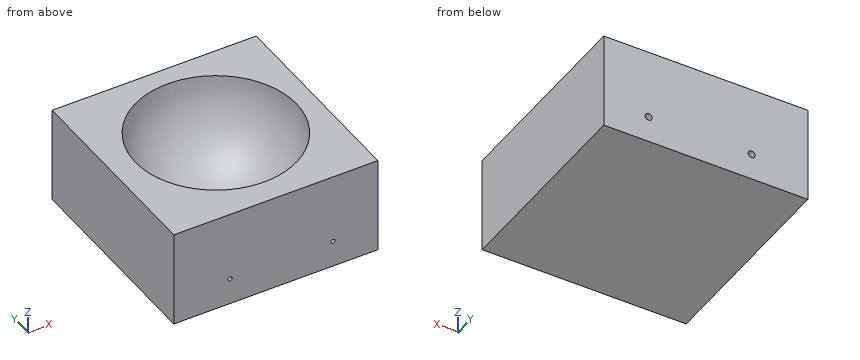
```python
from build123d import *

# Parameters (mm, degrees)
F0_W           = 190
F0_H           = 190
F1_DEPTH       = 90
F5_D           = 4
F5_CBORE_D     = 6.5
F5_CBORE_DEPTH = 50


with BuildPart() as f1:
    # F0 (on Top) → F1 (new body)
    with BuildSketch(Plane.XY):
        with Locations((-2.279991, -2.496977)):
            Rectangle(F0_W, F0_H)
    extrude(amount=F1_DEPTH)

    # F2 (on face) → F3 (revolve, cut)
    with BuildSketch(Plane.XY.offset(90)):
        with BuildLine():
            Line((75, 0), (-75, 0))
            ThreePointArc((-75, 0), (0, -75), (75, 0))
        make_face()
    revolve(axis=Axis((0, 0, 90), (1, 0, 0)), mode=Mode.SUBTRACT)

    # F5 (through all)
    with Locations(Plane(origin=(0, 92.503023, 0), x_dir=(-1, 0, 0), z_dir=(0, 1, 0))):
        with Locations((44.935185, 24.847355), (-50.961897, 24.847355)):
            CounterBoreHole(F5_D / 2, F5_CBORE_D / 2, F5_CBORE_DEPTH)


solid = f1.part
```
Source: CAD feature listing. Evaluate the final solid. Frame: model axes, mm. Give positions to 0.01 mm unless a question says otherwise; leave off trailing zeros. Loops run counter-clockwise (first coordinate to the right, second up) from the corner with the lowest first, then second, coordinate; pieces in that order, holes last. Notation, with made-up numbers: (36.5, -39.5) - (55.5, -39.5) arc R12 cw to (55.5, -25.5) - close; hole circle Ø11 at (14.25, -21). An arc over 180 degrees is marked (long way). Use CSV: the item, a comma, the result in double quotes. Start each with the question number.
1. Section B-B (z = 68). Output: boundary loops of the cut face in (x, y).
2. Ray query, L1, parallel to Z at x = 50, y = 22.5; L2, parallel to X at y = 56, z = 27; L3, parallel to X at y = -31, z = 52.5. Return the intervals inside material, ascending.
3. Section C-C (x = -35). Output: boundary loops of the cut face in (y, z) (1 decimal).
4. Section D-D (y = 51). Output: boundary loops of the cut face in (x, z).
5. Pin query (flat end, axial travel): pin 1 (5 mm diameter, centred on x = -44.94, z = 24.85, fed in from +Y); pin 2 (2 mm diameter, centred on x = -45.5, z = 24.5, fed in from +Y). Return the tip coordinate at first contact, or that it passes through.
6. Section A-A (y = -31). Output: boundary loops of the cut face in (x, z).
Response:
1,outline,"(-97.28, -97.5) - (92.72, -97.5) - (92.72, 92.5) - (-97.28, 92.5) - close; hole circle Ø143.4 at (0, 0)"
2,L1,"0 to 23.09, 26.6 to 38.83"
2,L2,"-97.28 to -47.37, -42.5 to 48.53, 53.4 to 92.72"
2,L3,"-97.28 to -57.08, 57.08 to 92.72"
3,outline,"(-97.5, 0) - (92.5, 0) - (92.5, 90) - (66.3, 90) arc R66.3 cw to (-66.3, 90) - (-97.5, 90) - close"
4,outline,"(-97.28, 0) - (92.72, 0) - (92.72, 90) - (54.99, 90) arc R54.99 cw to (-54.99, 90) - (-97.28, 90) - close; hole circle Ø6.5 at (-44.94, 24.85); hole circle Ø6.5 at (50.96, 24.85)"
5,pin 1,"y = 42.5"
5,pin 2,"through"
6,outline,"(-97.28, 0) - (92.72, 0) - (92.72, 90) - (68.29, 90) arc R68.29 cw to (-68.29, 90) - (-97.28, 90) - close; hole circle Ø4 at (-44.94, 24.85); hole circle Ø4 at (50.96, 24.85)"
